```python
from build123d import *

# Parameters (mm, degrees)
BOSS_EXTRUDE1_DEPTH = 4
SKETCH2_R           = 1.4
SKETCH2_R_2         = 1.425
SKETCH2_R_3         = 1
CUT_EXTRUDE1_DEPTH  = 96.117033175


with BuildPart() as part:
    # Sketch1 → Boss-Extrude1 (new body)
    with BuildSketch(Plane(origin=(0, 0, 0), x_dir=(1, 0, 0), z_dir=(0, 1, 0))):
        with BuildLine():
            Line((-42.260071937, -28.563309365), (-31.239928063, -54.436690635))
            ThreePointArc((-31.239928063, -54.436690635), (-31.060593954, -55.012366758), (-31, -55.61227683))
            Line((-31, -55.61227683), (-31, -84))
            ThreePointArc((-31, -84), (-30.707106781, -84.707106781), (-30, -85))
            Line((-30, -85), (30, -85))
            ThreePointArc((30, -85), (30.707106781, -84.707106781), (31, -84))
            Line((31, -84), (31, -55.61227683))
            ThreePointArc((31, -55.61227683), (31.060593954, -55.012366758), (31.239928063, -54.436690635))
            Line((31.239928063, -54.436690635), (42.260071937, -28.563309365))
            ThreePointArc((42.260071937, -28.563309365), (42.439406046, -27.987633242), (42.5, -27.38772317))
            Line((42.5, -27.38772317), (42.5, 25))
            ThreePointArc((42.5, 25), (41.621320344, 27.121320344), (39.5, 28))
            Line((39.5, 28), (-39.5, 28))
            ThreePointArc((-39.5, 28), (-41.621320344, 27.121320344), (-42.5, 25))
            Line((-42.5, 25), (-42.5, -27.38772317))
            ThreePointArc((-42.5, -27.38772317), (-42.439406046, -27.987633242), (-42.260071937, -28.563309365))
        make_face()
    extrude(amount=BOSS_EXTRUDE1_DEPTH)

    # Sketch2 → Cut-Extrude1 (cut, through all)
    with BuildSketch(Plane(origin=(0, 4, 0), x_dir=(1, 0, 0), z_dir=(0, 1, 0))):
        with Locations(Location((39, 24.5, 0), (0, 0, 270))):
            Circle(SKETCH2_R)
        with Locations(Location((-19, 24.5, 0), (0, 0, 270))):
            Circle(SKETCH2_R)
        with Locations(Location((-28.3, -82.3, 0), (0, 0, 270))):
            Circle(SKETCH2_R)
        with Locations(Location((28.3, -82.3, 0), (0, 0, 270))):
            Circle(SKETCH2_R)
        with Locations(Location((26.5, 16, 0), (0, 0, 270))):
            Circle(SKETCH2_R_2)
        with Locations(Location((0.65, 16, 0), (0, 0, 270))):
            Circle(SKETCH2_R_2)
        with Locations(Location((26.5, -41.35, 0), (0, 0, 270))):
            Circle(SKETCH2_R_2)
        with Locations(Location((0.65, -41.35, 0), (0, 0, 270))):
            Circle(SKETCH2_R_2)
        with Locations(Location((-15.35, 16, 0), (0, 0, 270))):
            Circle(SKETCH2_R_3)
        with Locations(Location((-27.75, 16, 0), (0, 0, 270))):
            Circle(SKETCH2_R_3)
        with Locations(Location((-15.35, -48.6, 0), (0, 0, 270))):
            Circle(SKETCH2_R_3)
        with Locations(Location((-27.75, -48.6, 0), (0, 0, 270))):
            Circle(SKETCH2_R_3)
    extrude(amount=-CUT_EXTRUDE1_DEPTH, mode=Mode.SUBTRACT)


solid = part.part
```
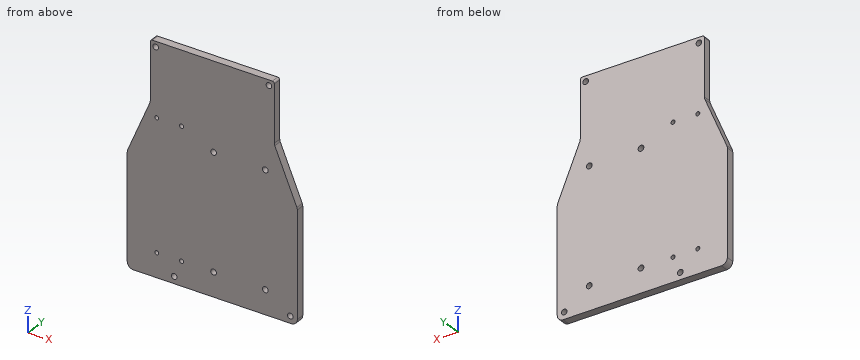
Geometry check sheet. Reference: the model listing, model coordinates, mm. Round coordinates to 2 decimals unless told otherwise and drop trailing zeros. Loops run counter-clockwise (first coordinate to the right, second up) from the corner with the lowest first, then second, coordinate; pieces in that order, holes last. Notation, with made-up numbers: (37, 84.25) -> (81, 84.25) arc R19 cw to (81, 91.25) -> close; hole circle Ø1 at (-39.5, 42.25). An arc over 180 degrees is marked (long way). Use a Markdown table: item, result.
(1) Scan lines: probe 1 along X at (y, z) = (1.3, -24.5); probe 2 along Z at (x, y) = (1.5, 3.75); probe 3 along Z at (x, y) = (-28.5, 2.15). Record each from-to range of solid material in increasing order.
Calculated:
| item | result |
|---|---|
| probe 1 | -42.5 to -20.4, -17.6 to 37.6, 40.4 to 42.5 |
| probe 2 | -28 to -17.14, -14.86 to 40.21, 42.49 to 85 |
| probe 3 | -28 to -16.66, -15.34 to 47.94, 49.26 to 80.91, 83.69 to 85 |
(2) Sectioned sample at A-A (x = -19). Enter the section's corners in (y, z).
Calculated:
| item | result |
|---|---|
| outline | (0, -28) -> (4, -28) -> (4, -25.9) -> (0, -25.9) -> close; (0, -23.1) -> (4, -23.1) -> (4, 85) -> (0, 85) -> close |
(3) Sectioned sample at B-B (x = 0.65). Enter the section's corners in (y, z) (3 decimals), then the cut area to 3 significant figures.
Calculated:
| item | result |
|---|---|
| outline | (0, -28) -> (4, -28) -> (4, -17.425) -> (0, -17.425) -> close; (0, -14.575) -> (4, -14.575) -> (4, 39.925) -> (0, 39.925) -> close; (0, 42.775) -> (4, 42.775) -> (4, 85) -> (0, 85) -> close |
| area | 429 mm² |
(4) Go/stop test with a flat-tipped pin: P1, Ø6, axis at x = 13.5, z = 56.5, coming from the -Y side. Record where the tip stops, or that it passes through.
Calculated:
| item | result |
|---|---|
| P1 | y = 0 |
(5) Sectioned sample at D-D (z = 41.35). Enter the section's corners in (x, y) (3 decimals), then the cut area to 3 significant figures.
Calculated:
| item | result |
|---|---|
| outline | (-36.814, 0) -> (-0.775, 0) -> (-0.775, 4) -> (-36.814, 4) -> close; (2.075, 0) -> (25.075, 0) -> (25.075, 4) -> (2.075, 4) -> close; (27.925, 0) -> (36.814, 0) -> (36.814, 4) -> (27.925, 4) -> close |
| area | 272 mm² |
(6) Sectioned sample at C-C (y = 3.35). Give the number of separate pieces and of enclosed holes in the cut face, then the cut area to 3 significant figures.
Calculated:
| item | result |
|---|---|
| separate pieces | 1 |
| enclosed holes | 12 |
| area | 8,540 mm² |
